For this review, take the finished solid that the model builds, in its own axes (mm). A direction names the side the tool comes from. Coordinates: 2 decimals unless noted, no trailing zeros. Loops run counter-clockwise (first coordinate to the right, second up) from the corner with the lowest first, then second, coordinate; pieces in that order, holes last. Notation, with made-up numbers: (32, 26) -> (38, 26) arc R9 cw to (38, 30) -> close; hole circle Ø4 at (-8, -2). An arc over 180 degrees is marked (long way). Answer in a Markdown table with one row per item.
from build123d import *

# Parameters (mm, degrees)
SKETCH1_R           = 5
SKETCH1_R_2         = 4
BOSS_EXTRUDE1_DEPTH = 5
FILLET3_R           = 5


with BuildPart() as part:
    # Sketch1 → Boss-Extrude1 (new body)
    with BuildSketch(Plane.XY):
        with BuildLine():
            Line((-10, 10), (10, 10))
            Line((10, 10), (10, -10))
            Line((10, -10), (-10, -10))
            ThreePointArc((-10, -10), (-80.710678119, 19.289321881), (-110, 90))
            Line((-110, 90), (-110, 170.890270731))
            Line((-110, 170.890270731), (-90, 170.890270731))
            Line((-90, 170.890270731), (-90, 90))
            ThreePointArc((-90, 90), (-89.793525108, 84.256016114), (-89.175166228, 78.541681939))
            Line((-89.175166228, 78.541681939), (-85.65069666, 80.144960069))
            ThreePointArc((-85.65069666, 80.144960069), (-72.859285644, 76.470042175), (-74.483275307, 63.260656311))
            Line((-74.483275307, 63.260656311), (-82.412785145, 55.994286547))
            ThreePointArc((-82.412785145, 55.994286547), (-52.892557185, 22.470535778), (-10, 10))
        make_face()
        Circle(SKETCH1_R, mode=Mode.SUBTRACT)
        with Locations((-100, 160.890270731)):
            Circle(SKETCH1_R_2, mode=Mode.SUBTRACT)
        with Locations((-81.407148813, 70.816413156)):
            Circle(SKETCH1_R, mode=Mode.SUBTRACT)
    extrude(amount=BOSS_EXTRUDE1_DEPTH)

    # Fillet3
    fillet3_edges = [part.edges().sort_by_distance(p)[0] for p in [
        (10, -10, 2.5),
        (-110, 170.890270731, 2.5),
        (-90, 170.890270731, 2.5),
        (10, 10, 2.5),
    ]]
    fillet(fillet3_edges, radius=FILLET3_R)


solid = part.part
Item 1: Take a section at B-B, the plane y = 0. State the section outline as (x, z) points, and give its area (3 significant figures).
Worked answers:
| item | result |
|---|---|
| outline | (-53.59, 0) -> (-5, 0) -> (-5, 5) -> (-53.59, 5) -> close; (5, 0) -> (10, 0) -> (10, 5) -> (5, 5) -> close |
| area | 268 mm² |
Item 2: Take a section at C-C, the plane z = 1.65. State the section outline as (x, y) points.
Worked answers:
| item | result |
|---|---|
| outline | (-110, 90) arc R100 ccw to (-10, -10) -> (5, -10) arc R5 ccw to (10, -5) -> (10, 5) arc R5 ccw to (5, 10) -> (-10, 10) arc R80 cw to (-82.41, 55.99) -> (-74.48, 63.26) arc R10.25 ccw to (-85.65, 80.14) -> (-89.18, 78.54) arc R80 cw to (-90, 90) -> (-90, 165.89) arc R5 ccw to (-95, 170.89) -> (-105, 170.89) arc R5 ccw to (-110, 165.89) -> close; hole circle Ø8 at (-100, 160.89); hole circle Ø10 at (-81.41, 70.82); hole circle Ø10 at (0, 0) |
Item 3: Take a section at D-D, the plane y = 142. State the section outline as (x, z) points, and give its area (4 significant figures).
Worked answers:
| item | result |
|---|---|
| outline | (-110, 0) -> (-90, 0) -> (-90, 5) -> (-110, 5) -> close |
| area | 100.0 mm² |
Item 4: The part is to be moulded in two halves that separate along Y. For faces 1 (the flat face through (-2, -10, 2)), 2 (the cylindrical face through (-108.57, 169.39, 2.54)), 3 (the cylindrical face through (-1.08, -4.88, 2.46)), say which applies: +Y half, -Y half, draft (parallel to the pull), parting line (faces both ways), or undercut.
Worked answers:
| item | result |
|---|---|
| face 1 | -Y half |
| face 2 | +Y half |
| face 3 | undercut |
Item 5: Take a section at A-A, the plane x = 0. State the section outline as (y, z) points.
Worked answers:
| item | result |
|---|---|
| outline | (-10, 0) -> (-5, 0) -> (-5, 5) -> (-10, 5) -> close; (5, 0) -> (10, 0) -> (10, 5) -> (5, 5) -> close |
Item 6: Insertion check: pin 1 (1 mm diameter, centred on y = 18.5, z = 1.5, fed in from +X); pin 2 (3 mm diameter, centred on x = -22.5, z = 4, fed in from +Y); pin 3 (1 mm diameter, centred on y = 18, z = 3.5, fed in from -X). Each pin has a flat end and moves straight along its axis. Give the tip position at first contact, or say it passes through.
Worked answers:
| item | result |
|---|---|
| pin 1 | x = -44.87 |
| pin 2 | y = 11.23 |
| pin 3 | x = -79.91 |
Item 7: For faces 4 (the flat face through (-90, 128, 2)), 5 (the flat face through (-100, 170.89, 2)), 6 (the cylindrical face through (-53.426, 22.812, 2.465)), list the 3-axis set-ups (+Z, -Z, +X, -X, +Y, -Y) from which the entire face can be reached by the end or side of a thin tool; tool diameter is ignored.
Worked answers:
| item | result |
|---|---|
| face 4 | +Z, -Z, +X, +Y |
| face 5 | +Z, -Z, +X, -X, +Y |
| face 6 | +Z, -Z, +X |
Item 8: For L1, parallel to Y at x = 0, z = 2.15; L2, parallel to Y at x = -99.5, z = 2.6; L3, parallel to X at y = 153, z = 4.15, list the stretches that pass through material, from the lowest coordinate up.
Worked answers:
| item | result |
|---|---|
| L1 | -10 to -5, 5 to 10 |
| L2 | 45.39 to 156.92, 164.86 to 170.89 |
| L3 | -110 to -90 |
